from build123d import *

# Parameters (mm, degrees)
ESBO_O1_W                = 68
ESBO_O1_H                = 53
RESSALTO_EXTRUS_O1_DEPTH = 2.5
ESBO_O2_R                = 3
ESBO_O2_R_2              = 1.3
RESSALTO_EXTRUS_O2_DEPTH = 2.5
FILETE1_R                = 4
CORTE_EXTRUS_O1_START    = -0.7
ESBO_O13_R               = 2.2
CORTE_EXTRUS_O1_DEPTH    = 43.479856415
ESBO_O14_R               = 1.3
CORTE_EXTRUS_O2_DEPTH    = 44.179856415
ESBO_O16_W               = 6
ESBO_O16_H               = 21
RESSALTO_EXTRUS_O4_DEPTH = 2.5
FILETE2_R                = 1


with BuildPart() as part:
    # Esboço1 → Ressalto-extrusão1 (new body)
    with BuildSketch(Plane.XY):
        Rectangle(ESBO_O1_W, ESBO_O1_H)
    extrude(amount=RESSALTO_EXTRUS_O1_DEPTH)

    # Esboço2 → Ressalto-extrusão2 (add)
    # profile 1 of 4: a face of its own
    with BuildSketch(Plane.XY.offset(2.5)):
        with Locations(Location((-28.5, 21, 0), (0, 0, 180))):
            Circle(ESBO_O2_R)
        with Locations((-28.5, 21)):
            Circle(ESBO_O2_R_2, mode=Mode.SUBTRACT)
    # profile 2 of 4: a face of its own
    with BuildSketch(Plane.XY.offset(2.5)):
        with Locations(Location((-28.5, -21, 0), (0, 0, 180))):
            Circle(ESBO_O2_R)
        with Locations(Location((-28.5, -21, 0), (0, 0, 180))):
            Circle(ESBO_O2_R_2, mode=Mode.SUBTRACT)
    # profile 3 of 4: a face of its own
    with BuildSketch(Plane.XY.offset(2.5)):
        with Locations(Location((28.5, -21, 0), (0, 0, 180))):
            Circle(ESBO_O2_R)
        with Locations((28.5, -21)):
            Circle(ESBO_O2_R_2, mode=Mode.SUBTRACT)
    # profile 4 of 4: a face of its own
    with BuildSketch(Plane.XY.offset(2.5)):
        with Locations(Location((28.5, 21, 0), (0, 0, 180))):
            Circle(ESBO_O2_R)
        with Locations(Location((28.5, 21, 0), (0, 0, 180))):
            Circle(ESBO_O2_R_2, mode=Mode.SUBTRACT)
    extrude(amount=RESSALTO_EXTRUS_O2_DEPTH)

    # Filete1
    filete1_edges = [part.edges().sort_by_distance(p)[0] for p in [
        (34, -26.5, 1.25),
        (-34, -26.5, 1.25),
        (-34, 26.5, 1.25),
        (34, 26.5, 1.25),
    ]]
    fillet(filete1_edges, radius=FILETE1_R)

    # Esboço13 → Corte-extrusão1 (cut, through all)
    with BuildSketch(Plane.XY.offset(2.5).offset(CORTE_EXTRUS_O1_START)):
        with Locations((-28.5, 21)):
            Circle(ESBO_O13_R)
        with Locations(Location((-28.5, -21, 0), (0, 0, 180))):
            Circle(ESBO_O13_R)
        with Locations((28.5, -21)):
            Circle(ESBO_O13_R)
        with Locations(Location((28.5, 21, 0), (0, 0, 180))):
            Circle(ESBO_O13_R)
    extrude(amount=-CORTE_EXTRUS_O1_DEPTH, mode=Mode.SUBTRACT)

    # Esboço14 → Corte-extrusão2 (cut, through all)
    with BuildSketch(Plane.XY.offset(2.5)):
        with Locations((-28.5, 21)):
            Circle(ESBO_O14_R)
        with Locations(Location((28.5, 21, 0), (0, 0, 180))):
            Circle(ESBO_O14_R)
        with Locations((28.5, -21)):
            Circle(ESBO_O14_R)
        with Locations(Location((-28.5, -21, 0), (0, 0, 180))):
            Circle(ESBO_O14_R)
    extrude(amount=-CORTE_EXTRUS_O2_DEPTH, mode=Mode.SUBTRACT)

    # Esboço16 → Ressalto-extrusão4 (add, through all)
    with BuildSketch(Plane.XY.offset(2.5)):
        with Locations((-37, 8)):
            Rectangle(ESBO_O16_W, ESBO_O16_H)
    extrude(amount=-RESSALTO_EXTRUS_O4_DEPTH)

    # Filete2
    filete2_edges = [part.edges().sort_by_distance(p)[0] for p in [
        (-34, 18.5, 1.25),
        (-34, -2.5, 1.25),
        (-40, -2.5, 1.25),
        (-40, 18.5, 1.25),
    ]]
    fillet(filete2_edges, radius=FILETE2_R)


solid = part.part
Can you work these out from the model? Positions are in its coordinate system, mm. A direction names the side the tool comes from. Give positions to 0.01 mm unless a question says otherwise; leave off trailing zeros. Write each loop counter-clockwise with the first axis right and the second up, starting at its lowest first coordinate (ties: lowest second). Pieces come first, ordered by that corner, then holes. Notation, with made-up numbers: M 68,62 L 81,62 A27 ccw 81,94 Z; hole C 59,71 d3. An arc over 180 degrees is marked long. Answer in a Markdown table with one row per item. Add a question column.
Item 1: Imagine slicing it at A-A, the plane y = 21. Write out the boundary of the cut face in (x, z), plus the area to 3 significant figures.
Item 2: Imagine slicing it at C-C, the plane x = -28.5. Write out the boundary of the cut face in (y, z), plus the area to 3 significant figures.
Item 3: Please list where these lines run through material, in increasing order: L1, parallel to Y at x = -28.5, z = 2.15; L2, parallel to Y at x = 28.5, z = 0.95; L3, parallel to Y at x = 28.5, z = 3.1.
Item 4: We'd pull the mould along Y, two halves only. Please class faces 4 (the flat face through (-37, 18.5, 1)), 5 (the cylindrical face through (31.5, -21.1, 3.7)), 6 (the flat face through (-4, 0, 0)): released by +Y, released by -Y, zero draft, split by the parting line, or undercut.
Item 5: Imagine slicing it at B-B, the plane z = 4.05. Write out the boundary of the cut face in (x, y).
Item 6: For pin 1 Ø3 at (y, z) = (5.5, 3) entering from +X; pin 2 Ø3.5 at (x, y) = (-28.5, 21) entering from -Z; pin 3 Ø12 at (x, y) = (-9, -9) entering from +Z; pin 4 Ø2 at (x, z) = (-37.5, 1.5) entering from +Y, each with a flat end and sliding along its axis, tell me the tip position at first contact or that it passes through.
Item 7: On a 3-axis mill with a long thin cutter (end or side, diameter ignored), from which of +Z, -Z, +X, -X, +Y, -Y can I reach the whole of each face in a straight line? I mean faces 1 (the flat face through (-4, 0, 2.5)), 2 (the flat face through (-34, 21, 1)), 3 (the cylindrical face through (26.754, -22.339, 0.913)). Say none if no direction works.
Item 8: Imagine slicing it at D-D, the plane y = -5. Write out the boundary of the cut face in (x, z), plus the area to 3 significant figures.
Evaluation:
| question | item | result |
|---|---|---|
| 1 | outline | M -34,0 L -30.7,0 L -30.7,1.8 L -29.8,1.8 L -29.8,5 L -31.5,5 L -31.5,2.5 L -34,2.5 Z; M -27.2,1.8 L -26.3,1.8 L -26.3,0 L 26.3,0 L 26.3,1.8 L 27.2,1.8 L 27.2,5 L 25.5,5 L 25.5,2.5 L -25.5,2.5 L -25.5,5 L -27.2,5 Z; M 29.8,1.8 L 30.7,1.8 L 30.7,0 L 34,0 L 34,2.5 L 31.5,2.5 L 31.5,5 L 29.8,5 Z |
| 1 | area | 168 mm² |
| 2 | outline | M -26.5,0 L -23.2,0 L -23.2,1.8 L -22.3,1.8 L -22.3,5 L -24,5 L -24,2.5 L -26.5,2.5 Z; M -19.7,1.8 L -18.8,1.8 L -18.8,0 L 18.8,0 L 18.8,1.8 L 19.7,1.8 L 19.7,5 L 18,5 L 18,2.5 L -18,2.5 L -18,5 L -19.7,5 Z; M 22.3,1.8 L 23.2,1.8 L 23.2,0 L 26.5,0 L 26.5,2.5 L 24,2.5 L 24,5 L 22.3,5 Z |
| 2 | area | 130 mm² |
| 3 | L1 | y = -26.5 to -22.3, -19.7 to 19.7, 22.3 to 26.5 |
| 3 | L2 | y = -26.5 to -23.2, -18.8 to 18.8, 23.2 to 26.5 |
| 3 | L3 | y = -24 to -22.3, -19.7 to -18, 18 to 19.7, 22.3 to 24 |
| 4 | face 4 | released by +Y |
| 4 | face 5 | undercut |
| 4 | face 6 | zero draft |
| 5 | outline | C -28.5,-21 d6; C -28.5,21 d6; C 28.5,-21 d6; C 28.5,21 d6; hole C -28.5,-21 d2.6; hole C -28.5,21 d2.6; hole C 28.5,-21 d2.6; hole C 28.5,21 d2.6 |
| 6 | pin 1 | stops at x = 34 |
| 6 | pin 2 | stops at z = 1.8 |
| 6 | pin 3 | stops at z = 2.5 |
| 6 | pin 4 | stops at y = 18.5 |
| 7 | face 1 | +Z |
| 7 | face 2 | +Z, -Z, -X, +Y |
| 7 | face 3 | -Z |
| 8 | outline | M -34,0 L 34,0 L 34,2.5 L -34,2.5 Z |
| 8 | area | 170 mm² |
